from build123d import *

# Parameters (mm, degrees)
SM_BASE_FLANGE_1_DEPTH = 1.2
SKETCH_5_R             = 3
CUT_EXTRUDE_1_DEPTH    = 64.494960298
OTHER_START            = 15.362016
OTHER_1_OUTLINE_W      = 70
OTHER_1_OUTLINE_H      = 1.2
OTHER_1_DEPTH          = 37.601839442
OTHER_START_2          = -52.963855442
OTHER_1_2_OUTLINE_W    = 70
OTHER_1_2_OUTLINE_H    = 1.2
OTHER_1_2_DEPTH        = 37.565871442
OTHER_START_3          = -15.7
OTHER_1_3_OUTLINE_R    = 3
OTHER_1_3_DEPTH        = 3.2
OTHER_START_4          = 12.5
OTHER_1_4_OUTLINE_R    = 3
OTHER_1_4_DEPTH        = 3.2
OTHER_START_5          = -35
OTHER_1_5_DEPTH        = 70


with BuildPart() as part:
    # 基体-法兰1: sheet metal written as solids
    # Sketch 1 → 基体-法兰1 (new body)
    with BuildSketch(Plane.XY):
        Polygon((35, 29.5), (28, 34.498419782), (28, 47.289071522), (23.238290906, 52.963855442), (-23.238290906, 52.963855442), (-28, 47.289071522), (-28, 34.498419782), (-35, 29.5), (-35, -29.5), (-28, -34.498419782), (-28, -47.289071522), (-23.238290906, -52.963855442), (23.238290906, -52.963855442), (28, -47.289071522), (28, -34.498419782), (35, -29.5), align=None)
    extrude(amount=-SM_BASE_FLANGE_1_DEPTH)

    # 草图5 → 切除-拉伸1 (cut, through all)
    with BuildSketch(Plane.XY):
        with Locations((-20, 43.963855442)):
            Circle(SKETCH_5_R)
        with Locations(Location((20, 43.963855442, 0), (0, 0, 180))):
            Circle(SKETCH_5_R)
        with Locations((20, -43.963855442)):
            Circle(SKETCH_5_R)
        with Locations(Location((-20, -43.963855442, 0), (0, 0, 180))):
            Circle(SKETCH_5_R)
    extrude(amount=-CUT_EXTRUDE_1_DEPTH, mode=Mode.SUBTRACT)

    # Other 1: read off the stored shape, not the designer's step
    # Other 1 outline → Other 1 (cut)
    with BuildSketch(Plane(origin=(0, 0, 0), x_dir=(1, 0, 0), z_dir=(0, 1, 0)).offset(OTHER_START)):
        with Locations((0, 0.6)):
            Rectangle(OTHER_1_OUTLINE_W, OTHER_1_OUTLINE_H)
    extrude(amount=OTHER_1_DEPTH, mode=Mode.SUBTRACT)

    # Other 1 2 outline → Other 1 2 (cut)
    with BuildSketch(Plane(origin=(0, 0, 0), x_dir=(1, 0, 0), z_dir=(0, 1, 0)).offset(OTHER_START_2)):
        with Locations((0, 0.6)):
            Rectangle(OTHER_1_2_OUTLINE_W, OTHER_1_2_OUTLINE_H)
    extrude(amount=OTHER_1_2_DEPTH, mode=Mode.SUBTRACT)

    # Other 1 3 outline → Other 1 3 (add)
    with BuildSketch(Plane(origin=(0, 0, 0), x_dir=(1, 0, 0), z_dir=(0, 1, 0)).offset(OTHER_START_3)):
        Polygon((35, 0), (-35, 0), (-35, -14.91592955), (-28, -19.914349333), (-28, -32.705001072), (-23.238290906, -38.379784993), (23.238290906, -38.379784993), (28, -32.705001072), (28, -19.914349333), (35, -14.91592955), align=None)
        with Locations((-20, -29.379784993)):
            Circle(OTHER_1_3_OUTLINE_R, mode=Mode.SUBTRACT)
        with Locations((20, -29.379784993)):
            Circle(OTHER_1_3_OUTLINE_R, mode=Mode.SUBTRACT)
    extrude(amount=OTHER_1_3_DEPTH)

    # Other 1 4 outline → Other 1 4 (add)
    with BuildSketch(Plane(origin=(0, 0, 0), x_dir=(1, 0, 0), z_dir=(0, 1, 0)).offset(OTHER_START_4)):
        Polygon((35, 0), (-35, 0), (-35, -14.91592955), (-28, -19.914349333), (-28, -32.705001072), (-23.238290906, -38.379784993), (23.238290906, -38.379784993), (28, -32.705001072), (28, -19.914349333), (35, -14.91592955), align=None)
        with Locations((-20, -29.379784993)):
            Circle(OTHER_1_4_OUTLINE_R, mode=Mode.SUBTRACT)
        with Locations((20, -29.379784993)):
            Circle(OTHER_1_4_OUTLINE_R, mode=Mode.SUBTRACT)
    extrude(amount=OTHER_1_4_DEPTH)

    # Other 1 5 outline → Other 1 5 (cut)
    with BuildSketch(Plane.YZ.offset(OTHER_START_5)):
        with BuildLine():
            Line((14.5, 2), (14.5, 38.379784993))
            Line((14.5, 38.379784993), (12.5, 38.379784993))
            Line((12.5, 38.379784993), (12.5, 0))
            ThreePointArc((12.5, 0), (13.914213562, 0.585786438), (14.5, 2))
        make_face()
        with BuildLine():
            Line((-12.5, 38.379784993), (-14.5, 38.379784993))
            Line((-14.5, 38.379784993), (-14.5, 2))
            ThreePointArc((-14.5, 2), (-13.914213562, 0.585786438), (-12.5, 0))
            Line((-12.5, 0), (-12.5, 38.379784993))
        make_face()
        with BuildLine():
            Line((-15.397984, -1.2), (-12.5, -1.2))
            ThreePointArc((-12.5, -1.2), (-14.7627417, -0.2627417), (-15.7, 2))
            Line((-15.7, 2), (-15.7, 0))
            Line((-15.7, 0), (-15.397984, 0))
            Line((-15.397984, 0), (-15.397984, -1.2))
        make_face()
        with BuildLine():
            ThreePointArc((15.7, 2), (14.7627417, -0.2627417), (12.5, -1.2))
            Line((12.5, -1.2), (15.362016, -1.2))
            Line((15.362016, -1.2), (15.362016, 0))
            Line((15.362016, 0), (15.7, 0))
            Line((15.7, 0), (15.7, 2))
        make_face()
    extrude(amount=OTHER_1_5_DEPTH, mode=Mode.SUBTRACT)


solid = part.part
Verification items for the finished model (mm, model axes). A direction names the side the tool comes from. Give positions to 0.01 mm unless a question says otherwise; leave off trailing zeros. Order: outer loops, then holes, each group sorted by start corner. A loop starts at its lowest first (then second) coordinate and runs counter-clockwise, first axis right, second up. Notation, with made-up numbers: M 76.5,28 L 113.5,28 A5 ccw 113.5,35 Z; hole C 10.5,52 d8. An arc over 180 degrees is marked long. Answer as a JSON object with one key per item and string values. Group by question number.
1) Cross-section at A-A (z = 23). Enter the section's corners in (x, y), then the cut area to 3 significant figures.
2) Scan lines: line 1 along Z through (x, y) = (-20, 15); line 2 along Y through (x, z) = (-2, 31.5); line 3 along Z through (x, y) = (11, 1). Record each from-to range of solid material in increasing order. Write a range as [from, to].
3) Depth check by flat-ended pin: pin 1 Ø6 at (y, z) = (12, 34.5) entering from +X; pin 2 Ø1.3 at (y, z) = (-15.5, 25.5) entering from +X; pin 3 Ø4 at (x, y) = (18.5, 4) entering from +Z. Enter the tip coordinate at first touch or a pass-through.
4) Access from +Z, -Z, +X, -X, +Y, -Y to the whole of each face (thin tool, end or side, straight path). Record for faces 1 (the face through (0, 14.5, 20)), 2 (the face through (0, -15.7, 20)).
5) Mould release check, pull along Z, two halves, no side actions. Record for faces 3 (the face through (0, 15, 0)), 4 (the face through (-20.391, 15.092, 26.405)), 5 (the face through (19.609, 15.092, 26.405)), 6 (the face through (31.45, -15.11, 17.45)): released by +Z, released by -Z, zero draft, split by the parting line, or undercut.
6) Cross-section at C-C (x = -4). Enter the section's corners in (y, z).
7) Cross-section at B-B (x = -20). Enter the section's corners in (y, z).
8) Cross-section at D-D (y = 1.5). Enter the section's corners in (x, z), then the cut area to 3 significant figures.
Result sheet:
{
 "1": {"outline": "M -28,-15.7 L 28,-15.7 L 28,-14.5 L -28,-14.5 Z; M -28,14.5 L 28,14.5 L 28,15.7 L -28,15.7 Z", "area": "134 mm2"},
 "2": {"line 1": "z = [0, 26.38], [32.38, 38.38]", "line 2": "y = [-15.7, -14.5], [14.5, 15.7]", "line 3": "z = [-1.2, 0]"},
 "3": {"pin 1": "stops at x = 27.89", "pin 2": "stops at x = 28", "pin 3": "stops at z = 0"},
 "4": {"face 1": "+Z, +X, -X", "face 2": "+Z, -Z, +X, -X, -Y"},
 "5": {"face 3": "released by -Z", "face 4": "undercut", "face 5": "undercut", "face 6": "released by +Z"},
 "6": {"outline": "M -15.7,2 A3.2 ccw -12.5,-1.2 L 12.5,-1.2 A3.2 ccw 15.7,2 L 15.7,38.38 L 14.5,38.38 L 14.5,2 A2 cw 12.5,0 L -12.5,0 A2 cw -14.5,2 L -14.5,38.38 L -15.7,38.38 Z"},
 "7": {"outline": "M -15.7,2 A3.2 ccw -12.5,-1.2 L 12.5,-1.2 A3.2 ccw 15.7,2 L 15.7,26.38 L 14.5,26.38 L 14.5,2 A2 cw 12.5,0 L -12.5,0 A2 cw -14.5,2 L -14.5,26.38 L -15.7,26.38 Z; M -15.7,32.38 L -14.5,32.38 L -14.5,38.38 L -15.7,38.38 Z; M 14.5,32.38 L 15.7,32.38 L 15.7,38.38 L 14.5,38.38 Z"},
 "8": {"outline": "M -35,-1.2 L 35,-1.2 L 35,0 L -35,0 Z", "area": "84.0 mm2"}
}
